Geometry check sheet. Reference: the model listing, model coordinates, mm. A direction names the side the tool comes from. Round coordinates to 2 decimals unless told otherwise and drop trailing zeros. Order: outer loops, then holes, each group sorted by start corner. A loop starts at its lowest first (then second) coordinate and runs counter-clockwise, first axis right, second up.
```python
from build123d import *

# Parameters (mm, degrees)
EXTRUDE_1_DEPTH = 2


with BuildPart() as part:
    # Model → 凸台-拉伸1 (new body)
    with BuildSketch(Plane.XY):
        with BuildLine():
            Line((287.664550766, 8.035001988), (23.914550766, 8.035001988))
            Line((23.914550766, 8.035001988), (20.879974458, 11.754816811))
            Line((20.879974458, 11.754816811), (22.08435013, 12.730101001))
            Line((22.08435013, 12.730101001), (16.425816067, 19.66638978))
            ThreePointArc((16.425816067, 19.66638978), (22.207201951, 19.598265756), (25.914550766, 24.035001988))
            Line((25.914550766, 24.035001988), (25.914550766, 14.035001988))
            Line((25.914550766, 14.035001988), (27.414546887, 14.035001988))
            Line((27.414546887, 14.035001988), (27.414546887, 24.035001988))
            ThreePointArc((27.414546887, 24.035001988), (30.343479076, 16.963934176), (37.414546887, 14.035001988))
            Line((37.414546887, 14.035001988), (63.414550766, 14.035001988))
            ThreePointArc((63.414550766, 14.035001988), (70.485618578, 16.963934176), (73.414550766, 24.035001988))
            Line((73.414550766, 24.035001988), (73.414550766, 14.035001988))
            Line((73.414550766, 14.035001988), (74.914546887, 14.035001988))
            Line((74.914546887, 14.035001988), (74.914546887, 24.035001988))
            ThreePointArc((74.914546887, 24.035001988), (77.843479076, 16.963934176), (84.914546887, 14.035001988))
            Line((84.914546887, 14.035001988), (108.664550766, 14.035001988))
            ThreePointArc((108.664550766, 14.035001988), (115.735618578, 16.963934176), (118.664550766, 24.035001988))
            Line((118.664550766, 24.035001988), (118.664550766, 14.035001988))
            Line((118.664550766, 14.035001988), (120.664546887, 14.035001988))
            Line((120.664546887, 14.035001988), (120.664546887, 24.035001988))
            ThreePointArc((120.664546887, 24.035001988), (123.593479076, 16.963934176), (130.664546887, 14.035001988))
            Line((130.664546887, 14.035001988), (145.914550766, 14.035001988))
            ThreePointArc((145.914550766, 14.035001988), (152.985618578, 16.963934176), (155.914550766, 24.035001988))
            Line((155.914550766, 24.035001988), (155.914550766, 14.035001988))
            Line((155.914550766, 14.035001988), (157.414546887, 14.035001988))
            Line((157.414546887, 14.035001988), (157.414546887, 24.035001988))
            ThreePointArc((157.414546887, 24.035001988), (160.343479076, 16.963934176), (167.414546887, 14.035001988))
            Line((167.414546887, 14.035001988), (210.914550766, 14.035001988))
            ThreePointArc((210.914550766, 14.035001988), (217.985618578, 16.963934176), (220.914550766, 24.035001988))
            Line((220.914550766, 24.035001988), (220.914550766, 14.035001988))
            Line((220.914550766, 14.035001988), (222.414550766, 14.035001988))
            Line((222.414550766, 14.035001988), (222.414550766, 24.035001988))
            ThreePointArc((222.414550766, 24.035001988), (225.343482954, 16.963934176), (232.414550766, 14.035001988))
            Line((232.414550766, 14.035001988), (275.664550766, 14.035001988))
            ThreePointArc((275.664550766, 14.035001988), (282.735618578, 16.963934176), (285.664550766, 24.035001988))
            Line((285.664550766, 24.035001988), (285.664550766, 14.035001988))
            Line((285.664550766, 14.035001988), (287.664550766, 14.035001988))
            Line((287.664550766, 14.035001988), (287.664550766, 8.035001988))
        make_face()
    extrude(amount=EXTRUDE_1_DEPTH)


solid = part.part
```
(1) Draft check along X on faces 3 (the flat face through (154, 13, 2)), 4 (the flat face through (19.295, 16.15, 0.986)), 5 (the cylindrical face through (70.41, 16.89, 0.99)). Enter one of: released by +X, released by -X, zero draft, split by the parting line, or undercut.
Returned:
face 3: zero draft
face 4: released by -X
face 5: undercut
(2) Sectioned sample at A-A, the plane x = 256.5. Record the cut outline in (y, z) (3 decimals), and give its area (3 significant figures).
Returned:
outline: (8.035, 0) - (14.035, 0) - (14.035, 2) - (8.035, 2) - close
area: 12.0 mm2
(3) Set-up check for faces 1 (the cylindrical face through (77.77, 17.04, 0.99)), 2 (the flat face through (154, 13, 0)): record each of +Z, -Z, +X, -X, +Y, -Y from which the full face is reachable in a straight line by a thin tool's end or side.
Returned:
face 1: +Z, -Z, +Y
face 2: -Z, +X, -X, +Y, -Y
(4) Depth check by flat-ended pin: P1, Ø1, axis at x = 53, z = 1, coming from the +Y side (3 decimals); P2, Ø1, axis at y = 17, z = 0.5, coming from the -X side; P3, Ø1, axis at y = 18.5, z = 1, coming from the -X side. Enter the tip coordinate at first touch or a pass-through.
Returned:
P1: stops at y = 14.035
P2: stops at x = 18.19
P3: stops at x = 16.97
(5) Material ranges on line 1 (Y direction, x = 245.5, z = 1.7) (3 decimals); line 2 (X direction, y = 11.75, z = 0.8); line 3 (X direction, y = 10, z = 0.8), recorded low to high.
Returned:
line 1: y = 8.035 to 14.035
line 2: x = 20.88 to 287.66
line 3: x = 22.31 to 287.66
